Design review of the part built by this model. Coordinates are the model's own, in mm. Give positions to 0.01 mm unless a question says otherwise; leave off trailing zeros. Order: outer loops, then holes, each group sorted by start corner. A loop starts at its lowest first (then second) coordinate and runs counter-clockwise, first axis right, second up.
```python
from build123d import *

# Parameters (mm, degrees)
F0_W     = 94.0536260605
F0_H     = 77.4676054716
F1_DEPTH = 25.4
F3_D     = 50.8
F4_R     = 5.08


with BuildPart() as f1:
    # F0 (on Front) → F1 (new body)
    with BuildSketch(Plane.XZ):
        with Locations((-22.8047668934, 18.0189460516)):
            Rectangle(F0_W, F0_H)
    extrude(amount=F1_DEPTH)

    # F3 (through all)
    with Locations(Plane.XZ.offset(25.4)):
        with Locations((-30.6195504963, 18.0068686604)):
            Hole(F3_D / 2)

    # F4
    f4_edges = [f1.edges().sort_by_distance(p)[0] for p in [
        (-22.804767, -25.4, -20.714857),
        (-69.83158, -25.4, 18.018946),
        (24.222046, -25.4, 18.018946),
        (-22.804767, -25.4, 56.752749),
        (-56.01955, -25.4, 18.006869),
        (24.222046, -12.7, 56.752749),
        (-69.83158, -12.7, 56.752749),
        (-22.804767, 0, 56.752749),
        (24.222046, -12.7, -20.714857),
        (24.222046, 0, 18.018946),
        (-69.83158, -12.7, -20.714857),
        (-22.804767, 0, -20.714857),
        (-69.83158, 0, 18.018946),
        (-56.01955, 0, 18.006869),
    ]]
    fillet(f4_edges, radius=F4_R)


solid = f1.part
```
1. Draft analysis for pull direction Z (two halves, no side actions). For faces 1 (the face through (-5.244, -12.593, 19.124)), 2 (the face through (5, -25.4, 18)), 3 (the face through (-68.38, -12.81, -19.19)), 4 (the face through (-22.218, -1.528, 55.304)), state which applies: pulls with the +Z half, pulls with the -Z half, needs draft (parallel to the pull), parting line crosses it, or undercut.
Recorded:
face 1: undercut
face 2: needs draft
face 3: pulls with the -Z half
face 4: pulls with the +Z half
2. For line 1 along Y through (x, z) = (-65, -4); line 2 along X through (y, z) = (-8, 27.5); line 3 along X through (y, z) = (-3, -1.5), list the stretches that pass through material, from the lowest coordinate up.
Recorded:
line 1: y = -25.39 to -0.01
line 2: x = -69.83 to -54.18, -7.06 to 24.22
line 3: x = -69.39 to -47.57, -13.66 to 23.78
3. Take a section at A-A (y = -2.25). State the section outline as (x, z) points.
Recorded:
outline: (-68.97, -15.63) arc R4.22 ccw to (-64.75, -19.85) - (19.14, -19.85) arc R4.22 ccw to (23.36, -15.63) - (23.36, 51.67) arc R4.22 ccw to (19.14, 55.89) - (-64.75, 55.89) arc R4.22 ccw to (-68.97, 51.67) - close; hole circle Ø52.52 at (-30.62, 18.01)
4. Take a section at B-B (y = -7.5). State the section outline as (x, z) points, then the cut area to 3 significant figures.
Recorded:
outline: (-69.83, -15.63) arc R5.08 ccw to (-64.75, -20.71) - (19.14, -20.71) arc R5.08 ccw to (24.22, -15.63) - (24.22, 51.67) arc R5.08 ccw to (19.14, 56.75) - (-64.75, 56.75) arc R5.08 ccw to (-69.83, 51.67) - close; hole circle Ø50.8 at (-30.62, 18.01)
area: 5,240 mm2
